```python
from build123d import *

# Parameters (mm, degrees)
SKETCH_1_W      = 100
SKETCH_1_H      = 190
SKETCH_1_R      = 3.525
SKETCH_1_R_2    = 3.535
SKETCH_1_R_3    = 2.5
PAD_DEPTH       = 6
SKETCH_R        = 2.5
SKETCH_R_2      = 2.322826
POCKET_DEPTH    = 6
SKETCH002_R     = 2.5
POCKET001_DEPTH = 6
SKETCH003_R     = 5
POCKET002_DEPTH = 6
SKETCH004_R     = 2.6
POCKET003_DEPTH = 6
FILLET_R        = 5
SKETCH005_R     = 8.25
POCKET004_DEPTH = 6
SKETCH006_R     = 2.5
POCKET005_DEPTH = 6


with BuildPart() as part:
    # Sketch_1 → Pad (new body)
    with BuildSketch(Plane.XY):
        with Locations((50, 95)):
            Rectangle(SKETCH_1_W, SKETCH_1_H)
        with Locations((15, 15)):
            Circle(SKETCH_1_R, mode=Mode.SUBTRACT)
        with Locations((50, 15)):
            Circle(SKETCH_1_R, mode=Mode.SUBTRACT)
        with Locations((85, 15)):
            Circle(SKETCH_1_R_2, mode=Mode.SUBTRACT)
        with Locations((16.629946, 115)):
            Circle(SKETCH_1_R_3, mode=Mode.SUBTRACT)
        with Locations((86.629946, 115)):
            Circle(SKETCH_1_R_3, mode=Mode.SUBTRACT)
    extrude(amount=PAD_DEPTH)

    # Sketch (on Face11 of Pad) → Pocket (cut)
    with BuildSketch(Plane.XY.offset(6)):
        with Locations((39.978905, 119.513016)):
            Circle(SKETCH_R)
        with Locations((60.032207, 119.416237)):
            Circle(SKETCH_R)
        with Locations((39.978905, 139.513016)):
            Circle(SKETCH_R_2)
        with Locations((39.978905, 159.513016)):
            Circle(SKETCH_R)
        with Locations((39.978905, 179.513016)):
            Circle(SKETCH_R)
        with Locations((59.978905, 179.358719)):
            Circle(SKETCH_R)
    extrude(amount=-POCKET_DEPTH, mode=Mode.SUBTRACT)

    # Sketch002 (on Face4 of Pocket) → Pocket001 (cut)
    with BuildSketch(Plane(origin=(0, 0, 0), x_dir=(1, 0, 0), z_dir=(0, 0, -1))):
        with Locations((42.987591, -54.983551)):
            Circle(SKETCH002_R)
        with Locations((42.978264, -74.953857)):
            Circle(SKETCH002_R)
    extrude(amount=-POCKET001_DEPTH, mode=Mode.SUBTRACT)

    # Sketch003 (on Face5 of Pocket001) → Pocket002 (cut)
    with BuildSketch(Plane.XY.offset(6)):
        with Locations((65.499825, 149.501081)):
            Circle(SKETCH003_R)
    extrude(amount=-POCKET002_DEPTH, mode=Mode.SUBTRACT)

    # Sketch004 (on Face5 of Pocket002) → Pocket003 (cut)
    with BuildSketch(Plane.XY.offset(6)):
        with Locations((89.073647, 173.068237)):
            Circle(SKETCH004_R)
        with Locations((89.069992, 125.98822)):
            Circle(SKETCH004_R)
    extrude(amount=-POCKET003_DEPTH, mode=Mode.SUBTRACT)

    # Fillet
    fillet_edges = [part.edges().sort_by_distance(p)[0] for p in [
        (0, 190, 3),
        (100, 190, 3),
    ]]
    fillet(fillet_edges, radius=FILLET_R)

    # Sketch005 (on Face5 of Fillet) → Pocket004 (cut)
    with BuildSketch(Plane.XY.offset(6)):
        with Locations((65.499825, 149.501081)):
            Circle(SKETCH005_R)
    extrude(amount=-POCKET004_DEPTH, mode=Mode.SUBTRACT)

    # Sketch006 (on Face5 of Pocket004) → Pocket005 (cut)
    with BuildSketch(Plane.XY.offset(6)):
        with Locations((65.499825, 162.501081)):
            Circle(SKETCH006_R)
        with Locations((65.499825, 136.501081)):
            Circle(SKETCH006_R)
    extrude(amount=-POCKET005_DEPTH, mode=Mode.SUBTRACT)


solid = part.part
```
The listing builds one solid part. Answer for the finished solid, in the listing's coordinates (mm). Coordinates: 2 decimals unless noted, no trailing zeros. Write each loop counter-clockwise with the first axis right and the second up, starting at its lowest first coordinate (ties: lowest second). Pieces come first, ordered by that corner, then holes. Notation, with made-up numbers: (33.25, 19) - (40.25, 19) arc R31 ccw to (40.25, 44) - close; hole circle Ø7 at (32, 66.25). An arc over 180 degrees is marked (long way). One line per item, written item: value.
1) Find section A-A (y = 15). Give the vertices of the cut face in (x, z) (3 decimals).
Geometry check:
outline: (0, 0) - (11.475, 0) - (11.475, 6) - (0, 6) - close; (18.525, 0) - (46.475, 0) - (46.475, 6) - (18.525, 6) - close; (53.525, 0) - (81.465, 0) - (81.465, 6) - (53.525, 6) - close; (88.535, 0) - (100, 0) - (100, 6) - (88.535, 6) - close
2) Each of these flat-tipped pins is pushed along its axis until it touches: pin 1 Ø8 at (x, y) = (50, 15) entering from +Z; pin 2 Ø4 at (x, y) = (60.03, 119.42) entering from +Z. Where does it stop, or does it pass through?
Geometry check:
pin 1: stops at z = 6
pin 2: passes through
3) Find section B-B (x = 50). Give the vertices of the cut face in (y, z) (3 decimals), and give its area (3 significant figures).
Geometry check:
outline: (0, 0) - (11.475, 0) - (11.475, 6) - (0, 6) - close; (18.525, 0) - (190, 0) - (190, 6) - (18.525, 6) - close
area: 1,100 mm2
4) For a pull along X with two mould halves and no side action, classify faces 1 (the cylindrical face through (98, 189, 3)), 2 (the cylindrical face through (91.554, 173.849, 3.042)), 3 (the flat face through (49, 96, 0)) as pulls with the +X half, pulls with the -X half, needs draft (parallel to the pull), parting line crosses it, or undercut.
Geometry check:
face 1: pulls with the +X half
face 2: undercut
face 3: needs draft
5) Consider line 1 along X through (y, z) = (126, 4.1); line 2 along Y through (x, z) = (64, 0.45); line 3 along Y through (x, z) = (84.5, 0.4). Determine where each line is inside the solid, lowest interval first. Write a range as from..to.
Geometry check:
line 1: x = 0..86.47, 91.67..100
line 2: y = 0..134.5, 138.5..141.39, 157.61..160.5, 164.5..190
line 3: y = 0..11.5, 18.5..113.69, 116.31..190
6) Find section C-C (y = 115). Give the vertices of the cut face in (x, z), and give its area (3 significant figures).
Geometry check:
outline: (0, 0) - (14.13, 0) - (14.13, 6) - (0, 6) - close; (19.13, 0) - (84.13, 0) - (84.13, 6) - (19.13, 6) - close; (89.13, 0) - (100, 0) - (100, 6) - (89.13, 6) - close
area: 540 mm2
7) Find section D-D (z = 2.65). Count the separate pieces of the cut face and the enclosed holes in it, and give its area (3 significant figures).
Geometry check:
separate pieces: 1
enclosed holes: 18
area: 18,400 mm2
